from build123d import *

# Parameters (mm, degrees)
F0_W     = 38.1
F0_H     = 38.1
F0_R     = 2.2225
F1_DEPTH = 3.175
F2_R     = 5.08
F3_W     = 6.35
F3_H     = 6.35
F4_DEPTH = 25.4
F5_R     = 2.54


with BuildPart() as f1:
    # F0 (on Top) → F1 (new body)
    with BuildSketch(Plane.XY):
        Rectangle(F0_W, F0_H)
        with Locations((-12.7, -12.7)):
            Circle(F0_R, mode=Mode.SUBTRACT)
        with Locations((12.7, -12.7)):
            Circle(F0_R, mode=Mode.SUBTRACT)
        with Locations((-12.7, 12.7)):
            Circle(F0_R, mode=Mode.SUBTRACT)
        with Locations((12.7, 12.7)):
            Circle(F0_R, mode=Mode.SUBTRACT)
    extrude(amount=F1_DEPTH)

    # F2
    f2_edges = [f1.edges().sort_by_distance(p)[0] for p in [
        (19.05, -19.05, 1.5875),
        (19.05, 19.05, 1.5875),
        (-19.05, -19.05, 1.5875),
        (-19.05, 19.05, 1.5875),
    ]]
    fillet(f2_edges, radius=F2_R)

    # F3 (on face) → F4 (cut)
    with BuildSketch(Plane.XY.offset(3.175)):
        with Locations((0, 15.875)):
            Rectangle(F3_W, F3_H)
    extrude(amount=-F4_DEPTH, mode=Mode.SUBTRACT)

    # F5
    f5_edges = [f1.edges().sort_by_distance(p)[0] for p in [
        (-3.175, 19.05, 1.5875),
        (3.175, 19.05, 1.5875),
    ]]
    fillet(f5_edges, radius=F5_R)


solid = f1.part
Input: part model. Units: mm. Frame: model coordinates. A direction names the side the tool comes from. Round coordinates to 2 decimals unless told otherwise and drop trailing zeros. Order: outer loops, then holes, each group sorted by start corner. A loop starts at its lowest first (then second) coordinate and runs counter-clockwise, first axis right, second up. Notation, with made-up numbers: (-29, 74) - (24, 74) arc R17 ccw to (24, 99) - close; hole circle Ø6 at (77.25, -3.75). An arc over 180 degrees is marked (long way). Answer as a JSON object with one key per item and string values. Group by question number.
(1) Material intervals for probe 1 along Y at (x, z) = (-12.7, 1.7); probe 2 along X at (y, z) = (16.5, 0.35) (3 decimals), sorted ascending. Write a range as from..to.
(2) Draft query along Y for faces 3 (the face through (0, 0, 0)), 4 (the face through (-14.464, 11.348, 1.565)), 5 (the face through (17.522, 17.601, 1.61)). Return one class per face: released by +Y, released by -Y, zero draft, split by the parting line, or undercut.
(3) Cut plane D-D (x = -0.5). Return loops of the section in (y, z) (3 decimals), then the cut area to 3 significant figures.
(4) Cut plane A-A (y = -12.7). Count the separate pieces of the cut face and the enclosed holes in it, then the cut area to 3 significant figures.
(5) Reachability of faces 1 (the face through (-3.939, 18.326, 1.565)), 2 (the face through (19.05, 0, 2)) from +Z, -Z, +X, -X, +Y, -Y: full face, straight path, thin tool, end or side. Return the list, or none.
Here are the results:
{
 "1": {"probe 1": "y = -19.05..-14.92, -10.48..10.48, 14.92..19.05", "probe 2": "x = -18.375..-3.175, 3.175..18.375"},
 "2": {"face 3": "zero draft", "face 4": "undercut", "face 5": "released by +Y"},
 "3": {"outline": "(-19.05, 0) - (12.7, 0) - (12.7, 3.175) - (-19.05, 3.175) - close", "area": "101 mm^2"},
 "4": {"separate pieces": "3", "enclosed holes": "0", "area": "92.7 mm^2"},
 "5": {"face 1": "+Z, -Z, +Y", "face 2": "+Z, -Z, +X, +Y, -Y"}
}
